Autodesk Fusion 360 part; units mm, degrees
sketch "Sketch1" plane through (0, 0, 0) normal (0, 1, 0) x (1, 0, 0)
  line L0 (0, -2) -> (0, 6)
  line L1 (-2.75, 0) -> (-2.575, -2)
  line L2 (-2.75, 0) -> (-1.325, 0)
  line L3 (0, 6) -> (-1.5, 6)
  line L4 (-1.5, 6) -> (-1.5, 1)
  line L5 (-1.5, 1) -> (-1.325, 0.3469)
  line L6 (-1.325, 0.3469) -> (-1.325, 0)
  line L7 (0, -2) -> (-2.575, -2)
  dimension "d13" = 5
  dimension "d14" = 5.5
  dimension "d18" = 3
  dimension "d56" = 6
  dimension "d65" = 15
  dimension "d67" = 2
  dimension "d71" = 2.65
  dimension "d77" = 1
revolve "Revolve1" add sketch "Sketch1" angle 360 about axis through (0, 0, 2) along (0, 0, -1) makes body 1
fillet "Fillet3" radius 0.2 1 edges at (-2.4008, 0.9312, 2) on bodies 1
fillet "Fillet2" radius 0.1 1 edges at (-1.2353, 0.4791, 0) on bodies 1
sketch "Sketch2" plane through (0, 0, 2) normal (0, 0, 1) x (1, 0, 0)
  line L0 (-0.35, 0.35) -> (-1.75, 0.35)
  line L1 (-1.75, 0.35) -> (-1.75, -0.35)
  line L2 (-1.75, -0.35) -> (-0.35, -0.35)
  line L3 (-0.35, -0.35) -> (-0.35, -1.75)
  line L4 (-0.35, -1.75) -> (0.35, -1.75)
  line L5 (0.35, -1.75) -> (0.35, -0.35)
  line L6 (0.35, -0.35) -> (1.75, -0.35)
  line L7 (1.75, -0.35) -> (1.75, 0.35)
  line L8 (1.75, 0.35) -> (0.35, 0.35)
  line L9 (0.35, 0.35) -> (0.35, 1.75)
  line L10 (0.35, 1.75) -> (-0.35, 1.75)
  line L11 (-0.35, 1.75) -> (-0.35, 0.35)
  dimension "d81" = 360
  dimension "d83" = 0.7
  dimension "d84" = 3.5
extrude "Extrude1" add sketch "Sketch2" against normal blind 0.86 separate body makes body 2
draft "Draft1" angle -30 neutral plane through (0, 0, 2) pull (0, 0, 1) 4 faces at (1.75, -0.1167, 1.7133) (0.1167, 1.75, 1.7133) (-1.75, 0.1167, 1.7133) (-0.1167, -1.75, 1.7133) on bodies 2
fillet "Fillet1" radius 0.7 4 edges at (-0.35, 0.35, 1.57) (-0.35, -0.35, 1.57) (0.35, -0.35, 1.57) (0.35, 0.35, 1.57) on bodies 2
combine "Combine1" operation cut target body 1 tool bodies 2
thread "Thread3" thread offset 0 thread length 10
equation "adsk_nomdia = 3.00 mm"
equation "adsk_nomlen = 6.00 mm"
equation "adsk_headdia = 5.50 mm"
equation "adsk_phildia = 3.50 mm"
equation "adsk_midfillet = 0.10 mm"
equation "adsk_phildepth = 0.86 mm"
equation "adsk_shnklen = 1.00 mm"
equation "adsk_thrang = 15 deg"
equation "adsk_headang = 5 deg"
equation "d13 = adsk_headang"
equation "d14 = adsk_headdia"
equation "d18 = adsk_nomdia"
equation "adsk_philwidth = 0.70 mm"
equation "d52 = adsk_midfillet"
equation "d56 = adsk_nomlen"
equation "d65 = adsk_thrang"
equation "d67 = adsk_headh"
equation "adsk_headh = 2.00 mm"
equation "adsk_pitch1 = 0.50 mm"
equation "adsk_shnkdia = adsk_nomdia - 0.7 * adsk_pitch1"
equation "d71 = adsk_shnkdia"
equation "adsk_headtoprad = adsk_headh * 0.1"
equation "d76 = adsk_headtoprad"
equation "d77 = adsk_shnklen"
equation "d83 = adsk_philwidth"
equation "d84 = adsk_phildia"
equation "d86 = adsk_philwidth"
properties part number "ISO 7048 - H - M3 x 6 Steel 4.6 Plain"
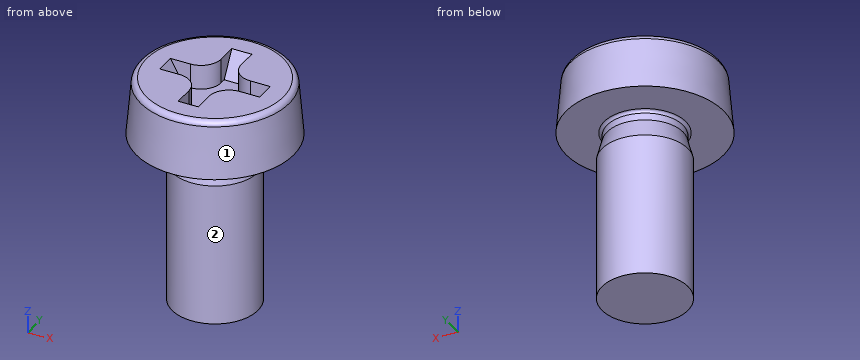
Could you check a few things on this model? Use its own coordinates, in mm. Face numbers are marked on the shaded views. A direction names the side the tool comes from. Coordinates: 2 decimals unless noted, no trailing zeros. Write each loop counter-clockwise with the first axis right and the second up, starting at its lowest first coordinate (ties: lowest second). Pieces come first, ordered by that corner, then holes. Notation, with made-up numbers: M 41.5,52.5 L 77.5,52.5 A8 cw 77.5,64.5 Z; hole C 19.25,64 d10. An arc over 180 degrees is marked long. Answer as CSV lines item,"result". Start each with the question number.
1) For the marked faces 1 and 2, which set-ups out of +Z, -Z, +X, -X, +Y, -Y let a thin tool reach every point of the face, with its end or its side?
2) I want a section at A-A, the plane y = 0. Please give me the cut outline in (x, z) (3 decimals).
3) I want a section at D-D, the plane z = 0.5. Please give me the cut outline in (x, y).
4) I want a section at C-C, the plane z = -1.25. Please give me the cut outline in (x, y), and give its area (3 significant figures).
5) Please list where these lines run through material, in increasing order: line 1 (Z direction, x = -1.05, y = -2.15); line 2 (Y direction, x = 0.15, z = 1.5). Write a range as from..to.
6) For P1, Ø0.8, axis at x = -1.5, z = 1.5, coming from the +Y side; P2, Ø0.6, axis at x = -1.5, z = 1.5, coming from the -Y side; P3, Ø2, axis at x = 0.5, y = 0.5, coming from the +Z side; P4, Ø3, axis at x = -2, z = -4.5, coming from the +Y side, each with a flat end and sliding along its axis, tell me the tip position at first contact or that it passes through.
Data:
1,face 1,"+Z"
1,face 2,"-Z"
2,outline,"M -2.75,0 L -1.425,0 A0.1 cw -1.325,-0.1 L -1.325,-0.347 L -1.5,-1 L -1.5,-6 L 1.5,-6 L 1.5,-1 L 1.325,-0.347 L 1.325,-0.1 A0.1 cw 1.425,0 L 2.75,0 L 2.591,1.817 A0.2 ccw 2.392,2 L 1.75,2 L 1.253,1.14 L -1.253,1.14 L -1.75,2 L -2.392,2 A0.2 ccw -2.591,1.817 Z"
3,outline,"C 0,0 d5.41"
4,outline,"C 0,0 d3"
4,area,"7.07 mm^2"
5,line 1,"z = 0..2"
5,line 2,"y = -2.61..-1.46, 1.46..2.61"
6,P1,"stops at y = 2.38"
6,P2,"stops at y = -2.33"
6,P3,"stops at z = 2"
6,P4,"stops at y = 1.41"
